Check sheet for the modelled part. Datum: model origin and axes. Units: mm. Give positions to 0.01 mm unless a question says otherwise; leave off trailing zeros. Write each loop counter-clockwise with the first axis right and the second up, starting at its lowest first coordinate (ties: lowest second). Pieces come first, ordered by that corner, then holes. Notation, with made-up numbers: (71.5, 43) -> (129.5, 43) arc R20 cw to (129.5, 54) -> close; hole circle Ø6 at (-12.5, 78.25). An arc over 180 degrees is marked (long way). Return JSON: item names as keys, results as strings.
Autodesk Fusion 360 part; units mm, degrees
sketch "スケッチ1" plane through (0, 0, 0) normal (0, 1, 0) x (1, 0, 0)
  line L0 (-140, 0) -> (-80, 0)
  line L1 (-80, 0) -> (-80, -4)
  line L2 (-80, -4) -> (-30, -4)
  line L3 (-30, -4) -> (-30, 0)
  line L4 (-30, 0) -> (30, 0)
  line L5 (30, 0) -> (30, -4)
  line L6 (30, -4) -> (80, -4)
  line L7 (80, -4) -> (80, 0)
  line L8 (80, 0) -> (140, 0)
  line L9 (140, 0) -> (140, 40)
  line L10 (140, 40) -> (80, 120)
  line L11 (80, 120) -> (-80, 120)
  line L12 (-80, 120) -> (-140, 40)
  line L13 (-140, 40) -> (-140, 0)
  line L14 (-57, 105) -> (57, 105)
  line L15 (75, 30) -> (115, 30)
  line L16 (-85, 35) -> (-85, 75)
  line L17 (-70, 110) -> (70, 110)
  line L18 (-130, 5) -> (130, 5)
  line L19 (-57, 105) -> (-57, 35)
  line L20 (-57, 35) -> (57, 35)
  line L21 (57, 105) -> (57, 35)
  line L22 (-58, 65) -> (58, 65)
  line L23 (58, 65) -> (58, 93)
  line L24 (58, 93) -> (-58, 93)
  line L25 (-58, 93) -> (-58, 65)
  point P0 (0, 120)
  point P1 (0, 105)
  point P2 (0, 110)
  point P3 (0, 5)
  point P4 (0, 65)
  dimension "d1" = 280
  dimension "d2" = 60
  dimension "d3" = 50
  dimension "d4" = 4
  dimension "d5" = 80
  dimension "d6" = 40
  dimension "d7" = 160
  dimension "d22" = 114
  dimension "d23" = 15
  dimension "d27" = 40
  dimension "d28" = 30
  dimension "d29" = 25
  dimension "d30" = 40
  dimension "d31" = 35
  dimension "d32" = 55
  dimension "d36" = 140
  dimension "d37" = 10
  dimension "d38" = 5
  dimension "d39" = 260
  dimension "d40" = 70
  dimension "d41" = 116
  dimension "d42" = 28
  dimension "d43" = 65
extrude "押し出し1" add sketch "スケッチ1" along normal blind 4 contours L0 L1 L2 L3 L4 L5 L6 L7 L8 L9 L10 L11 L12 L13 | L14 L19 L21 L24 | L19 L21 L22 L24 | L19 L22 L24 L25 | L21 L22 L23 L24 | L19 L20 L21 L22
hole "穴1" at (57, 0, -105) at (-57, 0, -105) at (-85, 0, -75) at (-85, 0, -35) at (75, 0, -30) at (115, 0, -30) at (-70, 0, -110) at (70, 0, -110) at (-130, 0, -5) at (130, 0, -5) at (-57, 0, -35) at (57, 0, -35) at (-58, 0, -93) at (-58, 0, -65) at (58, 0, -93) at (58, 0, -65) direction (0, 1, 0) diameter 3.2 end through all
sketch "スケッチ2" plane through (0, 4, 0) normal (0, 1, 0) x (-1, 0, 0)
  circle A0 centre (-58, -93) radius 1.6
  circle A1 centre (58, -93) radius 1.6
  circle A2 centre (57, -35) radius 1.6
  circle A3 centre (130, -5) radius 1.6
  circle A4 centre (70, -110) radius 1.6
  circle A5 centre (-75, -30) radius 1.6
  circle A6 centre (85, -75) radius 1.6
  circle A7 centre (-57, -105) radius 1.6
  circle A8 centre (57, -105) radius 1.6
  circle A9 centre (85, -35) radius 1.6
  circle A10 centre (-115, -30) radius 1.6
  circle A11 centre (-70, -110) radius 1.6
  circle A12 centre (-130, -5) radius 1.6
  circle A13 centre (-57, -35) radius 1.6
  circle A14 centre (58, -65) radius 1.6
  circle A15 centre (-58, -65) radius 1.6
  line L0 (140, -40) -> (140, 0)
  line L1 (140, 0) -> (80, 0)
  line L2 (80, 0) -> (80, 4)
  line L3 (80, 4) -> (30, 4)
  line L4 (30, 4) -> (30, 0)
  line L5 (30, 0) -> (-30, 0)
  line L6 (-30, 0) -> (-30, 4)
  line L7 (-30, 4) -> (-80, 4)
  line L8 (-80, 4) -> (-80, 0)
  line L9 (-80, 0) -> (-140, 0)
  line L10 (-140, 0) -> (-140, -40)
  line L11 (-140, -40) -> (-80, -120)
  line L12 (-80, -120) -> (80, -120)
  line L13 (80, -120) -> (140, -40)
  line L14 (68, -8) -> (42, -8)
  line L15 (42, -8) -> (42, -20)
  line L16 (42, -20) -> (68, -20)
  line L17 (68, -20) -> (68, -8)
  line L18 (-42, -8) -> (-68, -8)
  line L19 (-68, -8) -> (-68, -20)
  line L20 (-68, -20) -> (-42, -20)
  line L21 (-42, -20) -> (-42, -8)
  line L22 (83, -100) -> (65, -100)
  line L23 (65, -100) -> (65, -88)
  line L24 (65, -88) -> (83, -88)
  line L25 (83, -88) -> (83, -100)
  line L26 (55, 4) -> (55, -8)
  line L27 (-55, 4) -> (-55, -8)
  dimension "d44" = 18
  dimension "d45" = 12
  dimension "d46" = 12
  dimension "d47" = 88
  dimension "d48" = 65
  dimension "d50" = 26
extrude "押し出し2" cut sketch "スケッチ2" against normal through all contours L14 L15 L16 L17 | L18 L19 L20 L21 | L22 L23 L24 L25
(1) Cross-section at D-D on x = -100. Enter the section's corners in (y, z).
Reply:
{"outline": "(0, -93.33) -> (4, -93.33) -> (4, 0) -> (0, 0) -> close"}
(2) Cross-section at B-B on y = 1. State how many separate pieces and enclosed holes the cut face has, then the cut area to 3 significant figures.
Reply:
{"separate pieces": "1", "enclosed holes": "19", "area": "28,200 mm^2"}
(3) Cross-section at C-C on x = -4. Enter the section's corners in (y, z).
Reply:
{"outline": "(0, -120) -> (4, -120) -> (4, 0) -> (0, 0) -> close"}
(4) Cross-section at A-A on x = 50.5. Enter the section's corners in (y, z), then the cut area to 3 significant figures.
Reply:
{"outline": "(0, -120) -> (4, -120) -> (4, -20) -> (0, -20) -> close; (0, -8) -> (4, -8) -> (4, 4) -> (0, 4) -> close", "area": "448 mm^2"}
(5) Depth check by flat-ended pin: pin 1 Ø3 at (x, z) = (75, -30) entering from -Y (1 decimal); pin 2 Ø2 at (y, z) = (2, 1.5) entering from -X; pin 3 Ø2 at (x, y) = (112.5, 2.5) entering from +Z. Enter the tip coordinate at first touch or a pass-through.
Reply:
{"pin 1": "through", "pin 2": "x = -80", "pin 3": "z = 0"}
(6) Thickness scan on L1, parallel to X at y = 2.15, z = -35; L2, parallel to X at y = 1.85, z = -5; L3, parallel to Z at x = 51.5, y = 0.35. Record the ranges inside material, lowest first.
Reply:
{"L1": "-140 to -86.6, -83.4 to -58.6, -55.4 to 55.4, 58.6 to 140", "L2": "-140 to -131.6, -128.4 to 128.4, 131.6 to 140", "L3": "-120 to -20, -8 to 4"}
